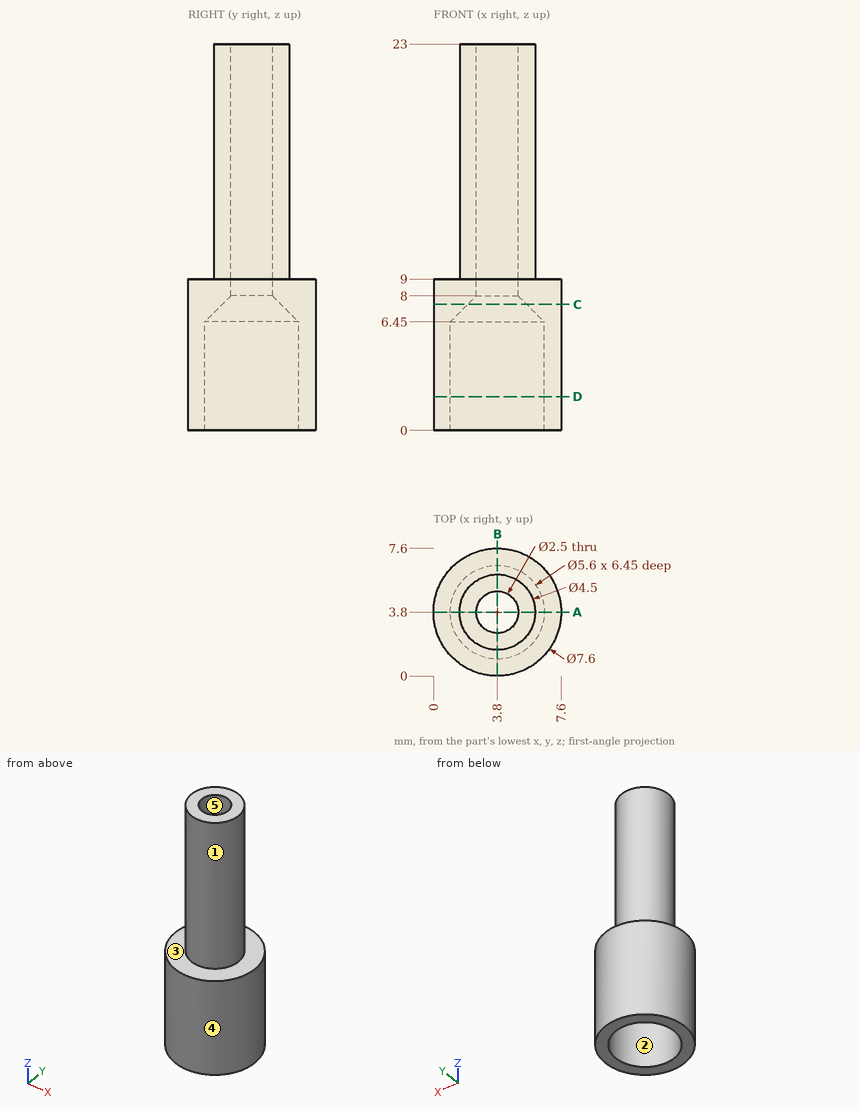
Source: three-view drawing plus pictorial views. Frame: mm from the lowest corner of the part. A direction names the side the tool comes from. Round coordinates to 2 decimals unless told otherwise and drop trailing zeros. Write each loop counter-clockwise with the first axis right and the second up, starting at its lowest first coordinate (ties: lowest second). Pieces come first, ordered by that corner, then holes. Notation, with made-up numbers: M 36,-34.75 L 51,-34.75 A6 ccw 51,-26.75 Z; hole C -38.75,24 d9. An arc over 180 degrees is marked long. One line per item, written item: value. Start each with the question number.
Item 1: Pin query (flat end, axial travel): pin 1 (1.5 mm diameter, centred on x = 3.8, y = 3.8, fed in from -Z); pin 2 (4 mm diameter, centred on y = 4.5, z = 16, fed in from +X); pin 3 (4.5 mm diameter, centred on x = 3.8, y = 3.8, fed in from -Z). Return the tip coordinate at first contact, or that it passes through.
Item 2: Set-up query: the marked faces 1 and 2. Return all of +Z, -Z, +X, -X, +Y, -Y with unobstructed straight access to the full face (end or side cutting, diameter ignored); none if empty.
Item 3: Mould query, pull axis Y, two halves, no side actions, for the marked faces 3, 4 and 5. Classes: pulls with the +Y half, pulls with the -Y half, needs draft (parallel to the pull), parting line crosses it, or undercut.
Item 4: Section query C-C (z = 7.5). Return the cut outline in (x, y), plus the area to 3 significant figures.
Item 5: Section query D-D (z = 2). Return the cut outline in (x, y).
Item 6: Section query A-A (y = 3.8). Return the cut outline in (x, z).
Item 7: Ray query, L1, parallel to Y at x = 3.8, z = 4; L2, parallel to Y at x = 3.8, z = 16.75; L3, parallel to Z at x = 5.5, y = 1.25. Return the intervals inside material, ascending. Write a range as from..to.
Result set:
1. pin 1: passes through
1. pin 2: stops at x = 6.05
1. pin 3: stops at z = 7
2. face 1: +Z
2. face 2: -Z
3. face 3: needs draft
3. face 4: parting line crosses it
3. face 5: undercut
4. outline: C 3.8,3.8 d7.6; hole C 3.8,3.8 d3.5
4. area: 35.7 mm²
5. outline: C 3.8,3.8 d7.6; hole C 3.8,3.8 d5.6
6. outline: M 0,0 L 1,0 L 1,6.45 L 2.55,8 L 2.55,23 L 1.55,23 L 1.55,9 L 0,9 Z; M 5.05,8 L 6.6,6.45 L 6.6,0 L 7.6,0 L 7.6,9 L 6.05,9 L 6.05,23 L 5.05,23 Z
7. L1: y = 0..1, 6.6..7.6
7. L2: y = 1.55..2.55, 5.05..6.05
7. L3: z = 0..9
